Can you work these out from the model? Positions are in its coordinate system, mm. Face numbers are marked on the shaded views. Round coordinates to 2 decimals unless told otherwise and drop trailing zeros. Order: outer loops, then holes, each group sorted by start corner. A loop starts at its lowest first (then second) coordinate and runs counter-clockwise, first axis right, second up. Notation, with made-up numbers: M -32,56.25 L -9,56.25 A19 cw -9,78.25 Z; hole C -19.5,72 d9. An arc over 180 degrees is marked long. Answer as a JSON object with one key per item and string values. Group by question number.
Autodesk Inventor part; units mm, degrees
ref_plane "YZ Plane" through (0, 0, 0) normal (1, 0, 0) x (0, 1, 0)
ref_plane "XZ Plane" through (0, 0, 0) normal (0, 1, 0) x (-1, 0, 0)
ref_plane "XY Plane" through (0, 0, 0) normal (0, 0, 1) x (1, 0, 0)
sketch "スケッチ1" plane through (0, 0, 0) normal (0, 0, 1) x (1, 0, 0)
  circle A0 centre (0, 0) radius 1.5
  dimension "d0" = 3
extrude "押し出し1" add sketch "スケッチ1" along normal blind 10
thread "ねじ1"
sketch "スケッチ2" plane through (0, 0, 10) normal (0, 0, 1) x (1, 0, 0)
  circle A0 centre (0, 0) radius 3
  dimension "d5" = 6
extrude "押し出し2" add sketch "スケッチ2" against normal blind 1.75
chamfer "面取り1" distance 1.5 angle 45 1 edges at (-3, 0, 8.25)
sketch "スケッチ3" plane through (0, 0, 10) normal (0, 0, 1) x (1, 0, 0)
  line L0 (0, 1.1547) -> (1, 0.5774)
  line L1 (1, 0.5774) -> (1, -0.5774)
  line L2 (1, -0.5774) -> (0, -1.1547)
  line L3 (0, -1.1547) -> (-1, -0.5774)
  line L4 (-1, -0.5774) -> (-1, 0.5774)
  line L5 (-1, 0.5774) -> (0, 1.1547)
  point P0 (0, 0)
  point P1 (0, 0)
  dimension "d11" = 2
extrude "押し出し3" cut sketch "スケッチ3" against normal blind 1.5
properties part number "m3皿ネジ10 (1)" material "鉄 灰色"
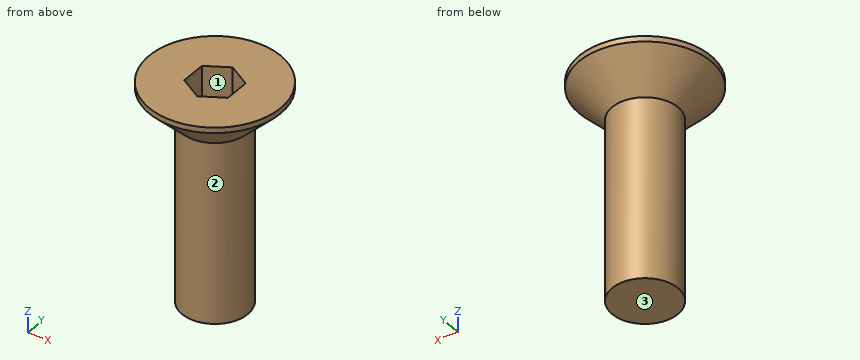
1) For pin 1 (0.6 mm diameter, centred on x = 0, y = 0, fed in from +Z); pin 2 (0.9 mm diameter, centred on y = 0, z = 9, fed in from +X); pin 3 (1.5 mm diameter, centred on x = -2, z = 1.5, fed in from +Y), each with a flat end and sliding along its axis, tell me the tip position at first contact or that it passes through.
2) If we section it at C-C on z = 6.5: Write out the boundary of the cut face in (x, y).
3) If we section it at A-A on z = 9: Write out the boundary of the cut face in (x, y).
4) We'd pull the mould along Y, two halves only. Please class the marked faces 1, 2 and 3: +Y half, -Y half, draft (parallel to the pull), parting line (faces both ways), or undercut.
5) I need wall thicknesses on line 1 along X through (y, z) = (-0.55, 7.5); line 2 along Z through (x, y) = (-0.05, 1.55); line 3 along Y through (x, z) = (0.15, 0.5). Which ranges of each line are inside material? Lowest first, please.
Findings:
{
 "1": {"pin 1": "stops at z = 8.5", "pin 2": "stops at x = 2.7", "pin 3": "stops at y = 0.83"},
 "2": {"outline": "C 0,0 d3"},
 "3": {"outline": "C 0,0 d4.5; hole M -1,-0.58 L 0,-1.15 L 1,-0.58 L 1,0.58 L 0,1.15 L -1,0.58 Z"},
 "4": {"face 1": "undercut", "face 2": "parting line", "face 3": "draft"},
 "5": {"line 1": "x = -1.4 to 1.4", "line 2": "z = 8.3 to 10", "line 3": "y = -1.49 to 1.49"}
}
